Work out the finished part from the listing and answer in its coordinate system (mm). Face numbers are marked on the shaded views. A direction names the side the tool comes from. Coordinates: 2 decimals unless noted, no trailing zeros. Order: outer loops, then holes, each group sorted by start corner. A loop starts at its lowest first (then second) coordinate and runs counter-clockwise, first axis right, second up. Notation, with made-up numbers: M 52.5,1 L 91.5,1 A21 cw 91.5,40 Z; hole C -31.5,38 d3. An arc over 180 degrees is marked long. Answer in a Markdown table with one row per item. Add a question column.
Item 1: Which of the six approach directions +Z, -Z, +X, -X, +Y, -Y give full straight-line access (tool end or side, diameter ignored) to the marked faces 1, 2 and 3?
Item 2: The mould has two halves that part along Y. Classify the marked faces 4, 5 and 6: released by +Y, released by -Y, zero draft, split by the parting line, or undercut.
Item 3: Consider line 1 (Y direction, x = 9, z = -0.5); line 2 (Y direction, x = 44, z = 10.5); line 3 (Y direction, x = 34.5, z = 17). Determine where each line is inside the solid, lowest interval first. Write a range as from..to.
Item 4: The part is cut by section A-A (x = 38). Write down the section's boundary in (y, z).
Item 5: The part is cut by section B-B (x = 62.5). Write down the section's boundary in (y, z), then the cut area to 3 significant figures.
Item 6: Flat-ended cylindrical pins translate along their axes: pin 1 Ø2 at (x, z) = (16.5, 14) entering from +Y; pin 2 Ø3 at (y, z) = (-3.5, -17) entering from +X; pin 3 Ø3 at (x, z) = (10.5, -6.5) entering from +Y; pin 4 Ø14.5 at (y, z) = (11.5, 9) entering from -X. Find the tip coordinate at first contact, or state that the pin passes through.
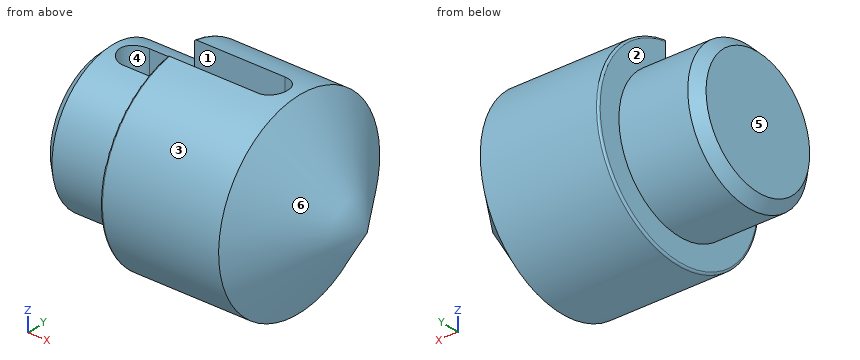
from build123d import *

# Parameters (mm, degrees)
F3_DEPTH = 25.4
F4_SIZE  = 2.54
F5_R     = 0.508


with BuildPart() as f1:
    # F0 (on Front) → F1 (revolve)
    with BuildSketch(Plane.XZ):
        Polygon((0, 18.442093), (0, 0), (67.2157, 0), (49.960807, 24.714644), (20, 24.714644), (20, 18.442093), align=None)
    revolve(axis=Axis((33.60785, 0, 0), (-1, 0, 0)))

    # F2 (on Top) → F3 (cut)
    with BuildSketch(Plane.XY):
        with BuildLine():
            Line((42.952237, 4.098997), (8.683674, 4.098997))
            ThreePointArc((8.683674, 4.098997), (4.584677, 0), (8.683674, -4.098997))
            Line((8.683674, -4.098997), (42.952237, -4.098997))
            ThreePointArc((42.952237, -4.098997), (47.051235, 0), (42.952237, 4.098997))
        make_face()
    extrude(amount=F3_DEPTH, mode=Mode.SUBTRACT)

    # F4
    f4_edges = [f1.edges().sort_by_distance(p)[0] for p in [
        (0, 0, -18.442093),
    ]]
    chamfer(f4_edges, length=F4_SIZE)

    # F5
    f5_edges = [f1.edges().sort_by_distance(p)[0] for p in [
        (20, 0, -24.714644),
    ]]
    fillet(f5_edges, radius=F5_R)


solid = f1.part
Reply:
| question | item | result |
|---|---|---|
| 1 | face 1 | +Z |
| 1 | face 2 | -X |
| 1 | face 3 | +X, -X |
| 2 | face 4 | undercut |
| 2 | face 5 | zero draft |
| 2 | face 6 | split by the parting line |
| 3 | line 1 | y = -18.44..18.44 |
| 3 | line 2 | y = -22.37..-3.96, 3.96..22.37 |
| 3 | line 3 | y = -17.94..-4.1, 4.1..17.94 |
| 4 | outline | M -4.1,0 L -4.1,24.37 A24.71 ccw long 4.1,24.37 L 4.1,0 Z |
| 5 | outline | C 0,0 d13.51 |
| 5 | area | 143 mm2 |
| 6 | pin 1 | stops at y = 13.08 |
| 6 | pin 2 | stops at x = 56.15 |
| 6 | pin 3 | stops at y = 17.75 |
| 6 | pin 4 | stops at x = 0 |
